Answer from the drawing. Dimensions are ordinates in mm from the lowest x, y and z of the part. A direction names the side the tool comes from. Coordinates: 2 decimals unless noted, no trailing zeros. Write each loop counter-clockwise with the first axis right and the second up, starting at its lowest first coordinate (ties: lowest second). Pieces come first, ordered by that corner, then holes. Notation, with made-up numbers: (-16.75, 4.25) -> (9.25, 4.25) arc R25 cw to (9.25, 38.25) -> close; hole circle Ø1 at (-18.75, -7). An arc over 180 degrees is marked (long way). Return JSON: item names as keys, results as strings.
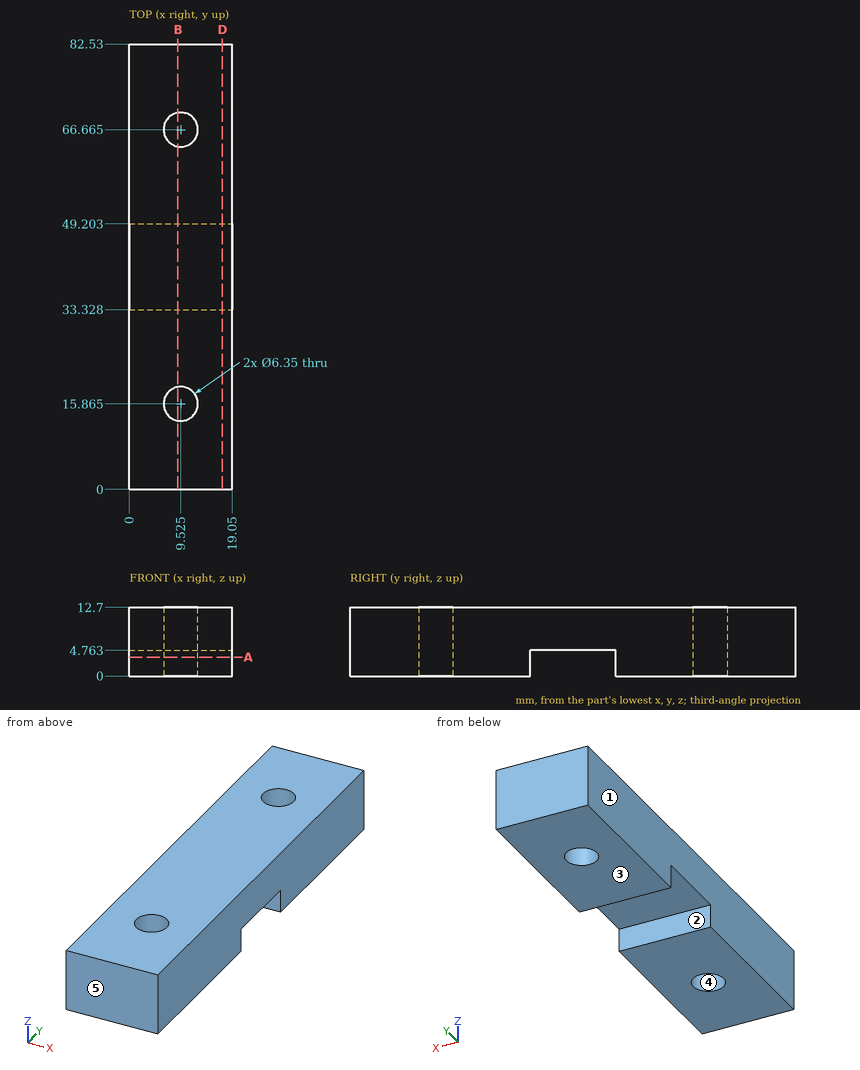
1. A tool of negligible diameter and unlimited length cuts with its end or side. For the marked faces 1 and 2, from which of +Z, -Z, +X, -X, +Y, -Y can it reach the whole face along a straight path? Write none if from no direction.
Taken from the geometry:
{"face 1": "+Z, -Z, -X, +Y, -Y", "face 2": "-Z, +X, -X"}
2. A flat-ended cylindrical pin translates along its axis: pin 1 Ø6 at (x, y) = (13, 44.5) entering from -Z. Find the tip coordinate at first contact, or state that the pin passes through.
Taken from the geometry:
{"pin 1": "stops at z = 4.76"}
3. The part is cut by section D-D (x = 17.25). Determine the outline of the cut face in (y, z).
Taken from the geometry:
{"outline": "(0, 0) -> (33.33, 0) -> (33.33, 4.76) -> (49.2, 4.76) -> (49.2, 0) -> (82.53, 0) -> (82.53, 12.7) -> (0, 12.7) -> close"}
4. The part is cut by section A-A (z = 3.5). Count the separate pieces of the cut face and the enclosed holes in it, then the cut area to 3 significant figures.
Taken from the geometry:
{"separate pieces": "2", "enclosed holes": "2", "area": "1,210 mm2"}
5. For a pull along Y with two mould halves and no side action, classify the marked faces 3, 4 and 5 as +Y half, -Y half, draft (parallel to the pull), parting line (faces both ways), or undercut.
Taken from the geometry:
{"face 3": "draft", "face 4": "undercut", "face 5": "-Y half"}
6. Consider L1, parallel to Y at x = 8, z = 7; L2, parallel to Y at x = 4.25, z = 1.25; L3, parallel to X at y = 16, z = 4.75. Determine where each line is inside the solid, lowest interval first.
Taken from the geometry:
{"L1": "y = 0 to 13.08, 18.65 to 63.88, 69.45 to 82.53", "L2": "y = 0 to 33.33, 49.2 to 82.53", "L3": "x = 0 to 6.35, 12.7 to 19.05"}
7. The part is cut by section B-B (x = 9). Determine the outline of the cut face in (y, z).
Taken from the geometry:
{"outline": "(0, 0) -> (12.73, 0) -> (12.73, 12.7) -> (0, 12.7) -> close; (19, 0) -> (33.33, 0) -> (33.33, 4.76) -> (49.2, 4.76) -> (49.2, 0) -> (63.53, 0) -> (63.53, 12.7) -> (19, 12.7) -> close; (69.8, 0) -> (82.53, 0) -> (82.53, 12.7) -> (69.8, 12.7) -> close"}
